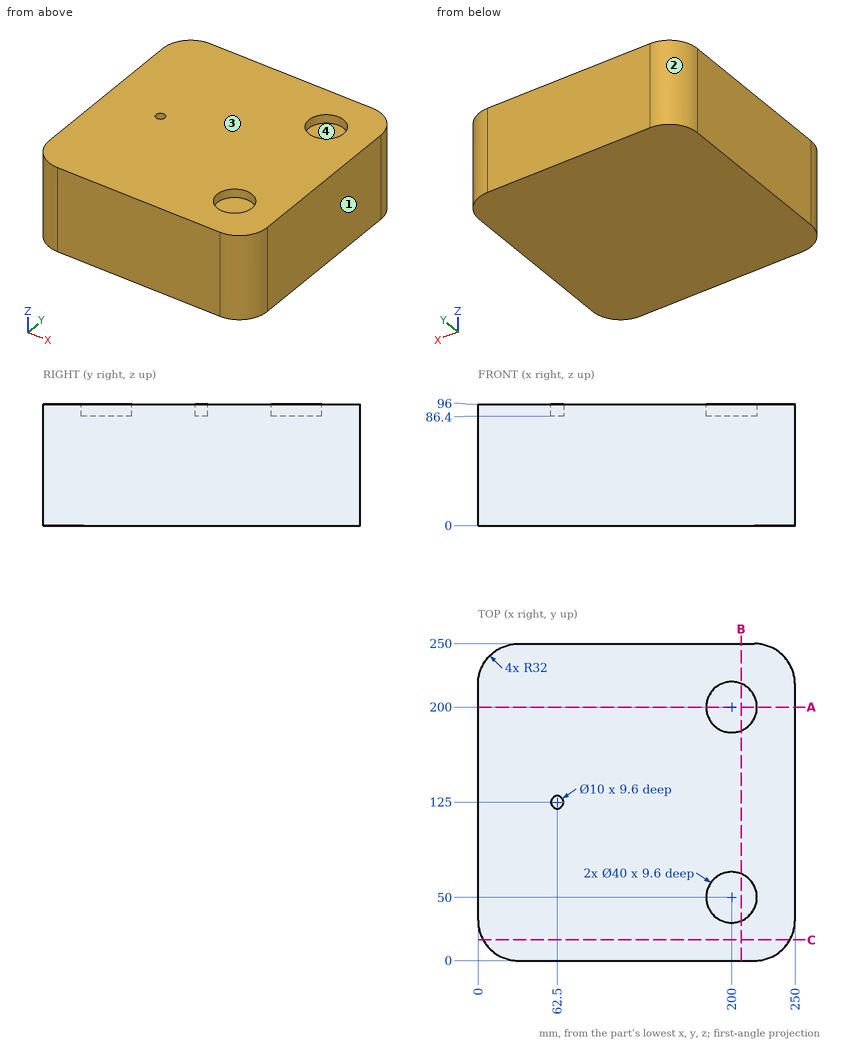
Answer from the drawing. Dimensions are ordinates in mm from the lowest x, y and z of the part. Round coordinates to 2 decimals unless told otherwise and drop trailing zeros. Write each loop counter-clockwise with the first axis right and the second up, starting at its lowest first coordinate (ties: lowest second). Pieces come first, ordered by that corner, then holes.
1. Determine the mould class of the marked faces 1, 2, 3 and 4 for opening direction X: pulls with the +X half, pulls with the -X half, needs draft (parallel to the pull), parting line crosses it, or undercut.
2. Given pin 1 Ø12 at (x, y) = (208.5, 44.5) entering from +Z, flat-ended and moving along its own axis, determine where the tip first touches the part or whether it passes through.
3. The part is cut by section C-C, the plane y = 16.5. Determine the outline of the cut face in (x, z).
4. The part is cut by section A-A, the plane y = 200. Determine the outline of the cut face in (x, z).
5. The part is cut by section B-B, the plane x = 207.5. Determine the outline of the cut face in (y, z).
6. A straight line is drawn through the part: L1, parallel to Y at x = 62, z = 91. Find the intervals that lie inside material, in ascending order.
Values:
1. face 1: pulls with the +X half
1. face 2: pulls with the -X half
1. face 3: needs draft
1. face 4: undercut
2. pin 1: stops at z = 86.4
3. outline: (4, 0) - (246, 0) - (246, 96) - (4, 96) - close
4. outline: (0, 0) - (250, 0) - (250, 96) - (220, 96) - (220, 86.4) - (180, 86.4) - (180, 96) - (0, 96) - close
5. outline: (0, 0) - (250, 0) - (250, 96) - (218.54, 96) - (218.54, 86.4) - (181.46, 86.4) - (181.46, 96) - (68.54, 96) - (68.54, 86.4) - (31.46, 86.4) - (31.46, 96) - (0, 96) - close
6. L1: y = 0 to 120.03, 129.97 to 250
